from build123d import *

# Parameters (mm, degrees)
SKETCH_1_W          = 100.539230484
SKETCH_1_H          = 40
SKETCH_1_W_2        = 17
SKETCH_1_H_2        = 7
EXTRUDE_1_DEPTH     = 2
SKETCH_2_W          = 100.539230484
SKETCH_2_H          = 40
SKETCH_2_R          = 2.25
EXTRUDE_2_DEPTH     = 1.5
SKETCH_3_W          = 184.808915215
SKETCH_3_H          = 94.825170589
CUT_EXTRUDE_1_DEPTH = 31.5
SKETCH_5_R          = 4
EXTRUDE_4_DEPTH     = 5
SKETCH_6_R          = 1.7
CUT_EXTRUDE_2_DEPTH = 10


with BuildPart() as part:
    # Эскиз1 → Бобышка-Вытянуть1 (new body)
    with BuildSketch(Plane.XY):
        with Locations((62.5, 12.5)):
            Rectangle(SKETCH_1_W, SKETCH_1_H)
        with Locations((24.230384758, 25)):
            Rectangle(SKETCH_1_W_2, SKETCH_1_H_2, mode=Mode.SUBTRACT)
        with Locations((100.769615242, 0)):
            Rectangle(SKETCH_1_W_2, SKETCH_1_H_2, mode=Mode.SUBTRACT)
    extrude(amount=EXTRUDE_1_DEPTH)

    # Эскиз2 → Бобышка-Вытянуть2 (add)
    with BuildSketch(Plane.XY.offset(2)):
        with Locations((62.5, 12.5)):
            Rectangle(SKETCH_2_W, SKETCH_2_H)
        with Locations((21.230384758, 25)):
            Circle(SKETCH_2_R, mode=Mode.SUBTRACT)
        with Locations((103.769615242, 0)):
            Circle(SKETCH_2_R, mode=Mode.SUBTRACT)
    extrude(amount=EXTRUDE_2_DEPTH)

    # Эскиз3 → Вырез-Вытянуть1 (cut)
    with BuildSketch(Plane.XY.offset(3.5)):
        with Locations((81.231416835, 7.831688581)):
            Rectangle(SKETCH_3_W, SKETCH_3_H)
        Polygon((12.230384758, 32.5), (42.230384758, 32.5), (54.020384758, 20.71), (75.769615242, 20.71), (88.979615242, 7.5), (112.769615242, 7.5), (112.769615242, -7.5), (82.769615242, -7.5), (66.982818678, 8.286796564), (45.230384758, 8.286796564), (36.017181322, 17.5), (12.230384758, 17.5), align=None, mode=Mode.SUBTRACT)
    extrude(amount=-CUT_EXTRUDE_1_DEPTH, mode=Mode.SUBTRACT)

    # Эскиз5 → Бобышка-Вытянуть4 (add)
    with BuildSketch(Plane.XY.offset(3.5)):
        with Locations((74.982818678, 14.5)):
            Circle(SKETCH_5_R)
    extrude(amount=EXTRUDE_4_DEPTH)

    # Эскиз6 → Вырез-Вытянуть2 (cut)
    with BuildSketch(Plane.XY.offset(8.5)):
        with Locations((74.982818678, 14.5)):
            Circle(SKETCH_6_R)
    extrude(amount=-CUT_EXTRUDE_2_DEPTH, mode=Mode.SUBTRACT)


solid = part.part
Could you check a few things on this model? Use its own coordinates, in mm. A direction names the side the tool comes from. Coordinates: 2 decimals unless noted, no trailing zeros. Loops run counter-clockwise (first coordinate to the right, second up) from the corner with the lowest first, then second, coordinate; pieces in that order, holes last.
1. For P1, Ø1.8, axis at x = 25.5, z = 2.5, coming from the -Y side; P2, Ø1, axis at x = 23, y = 24.5, coming from the +Z side; P3, Ø1, axis at y = 24.5, z = 1, coming from the +X side, each with a flat end and sliding along its axis, tell me the tip position at first contact or that it passes through.
2. For faces 4 (the face through (98, -7.5, 2)), 5 (the face through (101, 7.5, 2)), 6 (the face through (24, 17.5, 2)), 7 (the face through (24, 28.5, 1)), 8 (the face through (77, 15, 8.5)), which set-ups out of +Z, -Z, +X, -X, +Y, -Y let a thin tool reach every point of the face, with its end or its side?
3. Imagine slicing it at C-C (z = 4.75). Please give me the cut outline in (x, y).
4. We'd pull the mould along Y, two halves only. Please class faces 1 (the face through (101, -3.5, 1)), 2 (the face through (65, 20.71, 2)), 3 (the face through (72.03, 17.2, 5.96)): released by +Y, released by -Y, zero draft, split by the parting line, or undercut.
5. Imagine slicing it at A-A (y = 0). Please give me the cut outline in (x, z), and give its area (3 significant figures).
6. Imagine slicing it at D-D (x = 74.5). Please give me the cut outline in (y, z).
7. Imagine slicing it at B-B (x = 100). Please give me the cut outline in (y, z).
8. I need wall thicknesses on L1, parallel to Y at x = 98.5, z = 1.75; L2, parallel to Y at x = 61.5, z = 1.5; L3, parallel to Z at x = 96.5, y = -4.5. Which ranges of each line are inside material? Lowest first, please.
Computed values:
1. P1: stops at y = 17.5
1. P2: stops at z = 3.5
1. P3: stops at x = 50.73
2. face 4: +Z, -Z, +X, -X, -Y
2. face 5: +Z, -Z, +X, +Y
2. face 6: +Z, -Z, -X, -Y
2. face 7: -Z
2. face 8: +Z, +X, -X, +Y, -Y
3. outline: circle Ø8 at (74.98, 14.5); hole circle Ø3.4 at (74.98, 14.5)
4. face 1: undercut
4. face 2: released by +Y
4. face 3: split by the parting line
5. outline: (75.27, 0) - (92.27, 0) - (92.27, 2) - (101.52, 2) - (101.52, 3.5) - (75.27, 3.5) - close; (106.02, 2) - (109.27, 2) - (109.27, 0) - (112.77, 0) - (112.77, 3.5) - (106.02, 3.5) - close
5. area: 90.5 mm2
6. outline: (0.77, 0) - (12.87, 0) - (12.87, 8.5) - (10.53, 8.5) - (10.53, 3.5) - (0.77, 3.5) - close; (16.13, 0) - (20.71, 0) - (20.71, 3.5) - (18.47, 3.5) - (18.47, 8.5) - (16.13, 8.5) - close
7. outline: (-7.5, 0) - (-3.5, 0) - (-3.5, 2) - (3.5, 2) - (3.5, 0) - (7.5, 0) - (7.5, 3.5) - (-7.5, 3.5) - close
8. L1: y = -7.5 to -3.5, 3.5 to 7.5
8. L2: y = 8.29 to 20.71
8. L3: z = 0 to 3.5
